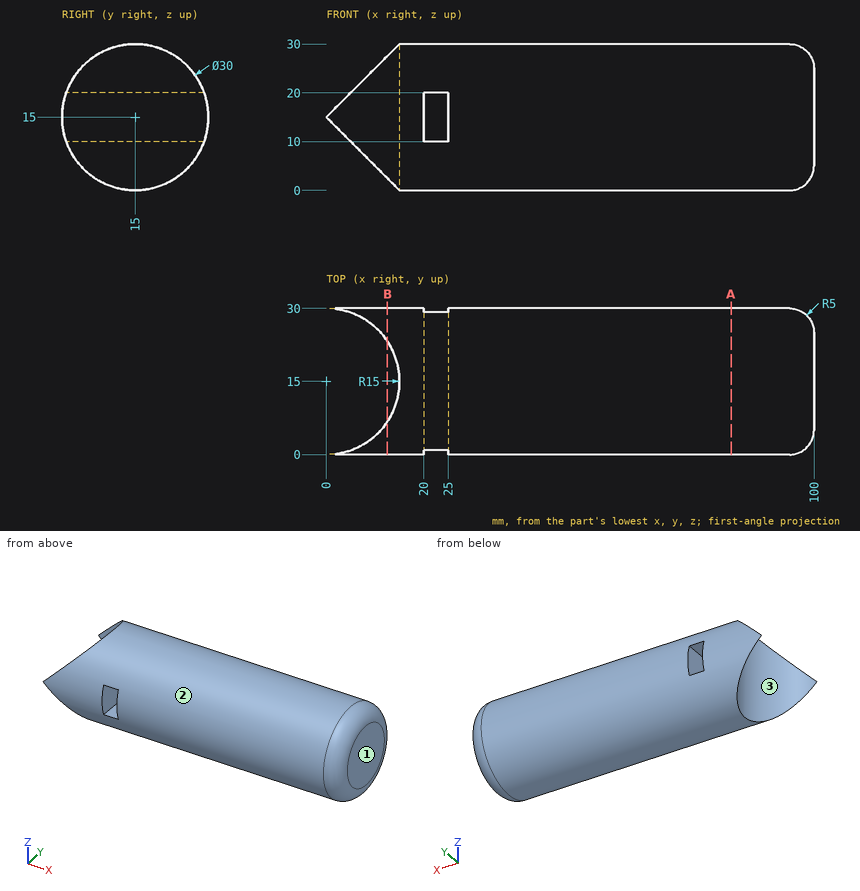
Geometry check sheet. Reference: drawing and pictorial views, mm from the part's lowest x, y, z. Coordinates: 2 decimals unless noted, no trailing zeros. Loops run counter-clockwise (first coordinate to the right, second up) from the corner with the lowest first, then second, coordinate; pieces in that order, holes last. Notation, with made-up numbers: (-34.75, 38) - (2.25, 38) arc R11 ccw to (2.25, 50) - close; hole circle Ø6 at (27.5, 71.5). An arc over 180 degrees is marked (long way). Return JSON: item names as keys, results as strings.
1. Section check A-A, the plane x = 83. Record the boundary of the cut face in (y, z).
Established:
{"outline": "circle Ø30 at (15, 15)"}
2. Go/stop test with flat-tipped pins: pin 1 (3 mm diameter, centred on y = 6, z = 4, fed in from -X); pin 2 (1.5 mm diameter, centred on x = 23, y = 18.5, fed in from -Z); pin 3 (4 mm diameter, centred on x = 23, y = 11.5, fed in from +Z). Record where each tip stops, or that it passes through.
Established:
{"pin 1": "stops at x = 10.74", "pin 2": "stops at z = 0.25", "pin 3": "stops at z = 29.92"}
3. Section check B-B, the plane x = 12.5. Record the boundary of the cut face in (y, z), then the cut area to 3 significant figures.
Established:
{"outline": "(6.71, 2.5) - (6.71, 27.5) arc R15 ccw to start; (23.29, 2.5) arc R15 ccw to (23.29, 27.5) - close", "area": "236 mm2"}
4. Thickness scan on L1, parallel to X at y = 28.5, z = 13.5; L2, parallel to X at y = 20.5, z = 11; L3, parallel to Z at x = 72, y = 10. Record the ranges inside material, lowest first.
Established:
{"L1": "x = 6.54 to 20, 25 to 98.49", "L2": "x = 13.96 to 20, 25 to 100", "L3": "z = 0.86 to 29.14"}
5. Mould release check, pull along Y, two halves, no side actions. Record for the marked faces 1, 2 and 3: +Y half, -Y half, draft (parallel to the pull), parting line (faces both ways), or undercut.
Established:
{"face 1": "draft", "face 2": "parting line", "face 3": "undercut"}
